Read the model definition and answer for the solid it produces. Units are mm, in the model's axes. A direction names the side the tool comes from. Give positions to 0.01 mm unless a question says otherwise; leave off trailing zeros. Write each loop counter-clockwise with the first axis right and the second up, starting at its lowest first coordinate (ties: lowest second). Pieces come first, ordered by that corner, then holes. Notation, with made-up numbers: (60, -37.5) - (66, -37.5) arc R19 ccw to (66, -12.5) - close; hole circle Ø2 at (-16.75, -20). An arc over 180 degrees is marked (long way). Answer as CSV lines item,"result".
Autodesk Inventor part; units mm, degrees
ref_plane "YZ Plane" through (0, 0, 0) normal (1, 0, 0) x (0, 1, 0)
ref_plane "XZ Plane" through (0, 0, 0) normal (0, 1, 0) x (-1, 0, 0)
ref_plane "XY Plane" through (0, 0, 0) normal (0, 0, 1) x (1, 0, 0)
sketch "Sketch1" plane through (0, 0, 0) normal (0, 1, 0) x (-1, 0, 0)
  line L0 (300, 200) -> (-300, 200)
  line L1 (-300, 200) -> (-300, -200)
  line L2 (-300, -200) -> (300, -200)
  line L3 (300, -200) -> (300, 200)
  line L4 (300, 200) -> (-300, -200) construction
  line L5 (-300, 200) -> (300, -200) construction
  line L6 (320, 220) -> (-320, 220)
  line L7 (-320, 220) -> (-320, 200)
  line L8 (-300, -220) -> (320, -220)
  line L9 (320, -220) -> (320, 220)
  line L10 (320, 220) -> (-320, -220) construction
  line L11 (-320, 220) -> (320, -220) construction
  line L12 (-300, -200) -> (-300, -220)
  line L13 (-300, 200) -> (-300, 220)
  point P0 (0, 0)
  dimension "d0" = 600
  dimension "d1" = 400
  dimension "d2" = 640
  dimension "d3" = 440
extrude "Extrusion1" add sketch "Sketch1" against normal blind 600 contours L0 L13 L6 L9 L8 L12 L2 L3
sketch "Sketch2" plane through (0, -600, 0) normal (0, -1, 0) x (1, 0, 0)
  line L0 (-320, -220) -> (-320, 220)
  line L1 (-320, -220) -> (300, -220)
  line L2 (300, -220) -> (300, 820)
  line L3 (300, 820) -> (-320, 820)
  line L4 (-320, 820) -> (-320, -220)
  point P0 (300, 220)
  point P1 (-320, 220)
  dimension "d14" = 1040
  dimension "d15" = 620
extrude "Extrusion2" add sketch "Sketch2" along normal blind 10
properties part number "Stage" material "Wood (Cherry)"
(1) Find the intervals of material crossed by L1, parallel to Z at x = -162.5, y = -328; L2, parallel to Y at x = -220, z = 773; L3, parallel to X at y = -213, z = -156.5, in increasing order.
Worked out:
L1,"z = -220 to -200, 200 to 220"
L2,"y = -610 to -600"
L3,"x = -320 to -300"
(2) The mould has two halves that part along Z. Classify faces 1 (the flat face through (-6, -301, -220)), 2 (the flat face through (-300, -296, -3)), 3 (the flat face through (300, -304, -203)): +Z half, -Z half, draft (parallel to the pull), parting line (faces both ways), or undercut.
Worked out:
face 1,"-Z half"
face 2,"undercut"
face 3,"draft"
(3) A cutting plane is placed at A-A (x = 231.5). Write down the section's boundary in (y, z), and give its area (3 significant figures).
Worked out:
outline,"(-610, -220) - (0, -220) - (0, -200) - (-600, -200) - (-600, 200) - (0, 200) - (0, 220) - (-600, 220) - (-600, 820) - (-610, 820) - close"
area,"34,400 mm^2"
(4) A cutting plane is placed at D-D (z = 403). Write down the section's boundary in (x, y).
Worked out:
outline,"(-320, -610) - (300, -610) - (300, -600) - (-320, -600) - close"
(5) A cutting plane is placed at B-B (y = -379). Write down the section's boundary in (x, z).
Worked out:
outline,"(-320, -220) - (300, -220) - (300, -200) - (-300, -200) - (-300, 200) - (300, 200) - (300, 220) - (-320, 220) - close"
(6) A cutting plane is placed at C-C (z = -61). Write down the section's boundary in (x, y), and give its area (3 significant figures).
Worked out:
outline,"(-320, -610) - (300, -610) - (300, -600) - (-300, -600) - (-300, 0) - (-320, 0) - close"
area,"18,200 mm^2"
(7) For faces 4 (the flat face through (-320, -301, -54)), 5 (the flat face through (-4, -296, 200)), 6 (the flat face through (-14, -296, 220)), determine the directions among +Z, -Z, +X, -X, +Y, -Y from which every point of the face is accessible in a straight line to the end or side of a thin tool.
Worked out:
face 4,"+Z, -Z, -X, +Y, -Y"
face 5,"+X, +Y"
face 6,"+Z, +X, -X, +Y"
(8) This flat-tipped pin is pushed along its axis until it touches: P1, Ø5, axis at x = 64, y = -222, coming from the +Z side. Where does it stop, or does it pass through?
Worked out:
P1,"stops at z = 220"
